Here's the drawing with two shaded views (mm, measured from the low corner). I have some questions. A direction names the side the tool comes from. Give positions to 0.01 mm unless a question says otherwise; leave off trailing zeros. Write each loop counter-clockwise with the first axis right and the second up, starting at its lowest first coordinate (ties: lowest second). Pieces come first, ordered by that corner, then holes. Notation, with made-up numbers: (1, -13.5) - (30, -13.5) arc R35 cw to (30, 22.5) - close; hole circle Ø10 at (0.5, 68). An arc over 180 degrees is marked (long way). Answer as a JSON object with one key per item and string values. Group by question number.
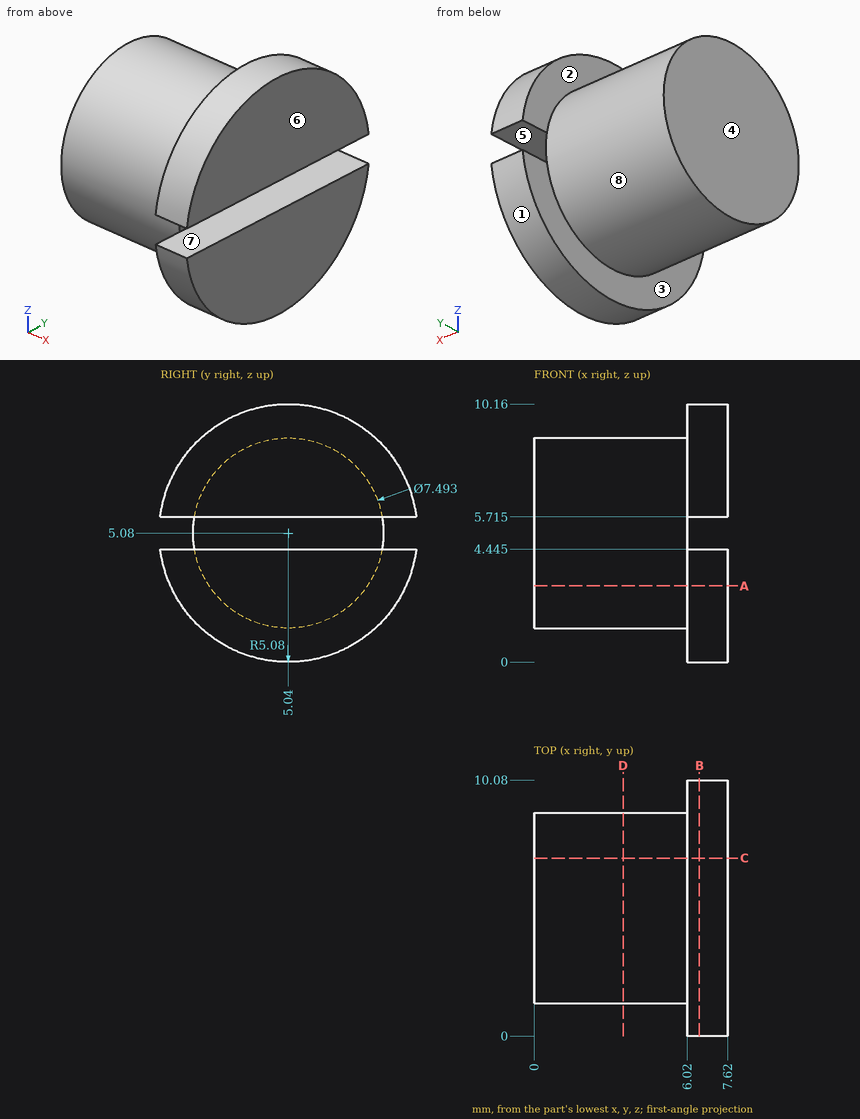
(1) I want a section at C-C, the plane y = 7. Please give me the cut outline in (x, z) (1 decimal), and give its area (3 significant figures).
(2) I want a section at D-D, the plane x = 3.5. Please give me the cut outline in (y, z), and give its area (3 significant figures).
(3) If we mould it in two halves opening along Z, with no side actions, what happens to the marked faces 6, 7 and 8? For each: +Z half, -Z half, draft (parallel to the pull), parting line (faces both ways), or undercut.
(4) Will these pins go through, and if not, where does the flat tip stop? P1, Ø3, axis at x = 6.5, y = 8, coming from the -Z side; P2, Ø3.5, axis at y = 7, z = 7.5, coming from the -X side; P3, Ø1.5, axis at x = 5, y = 4, coming from the -Z side (1 decimal); P4, Ø0.5, axis at x = 6.5, y = 6, coming from the -Z side.
(5) For the marked faces 1, 2, 3, 4 and 5, which set-ups out of +Z, -Z, +X, -X, +Y, -Y let a thin tool reach every point of the face, with its end or its side?
(6) I need wall thicknesses on L1, parallel to X at y = 2, z = 8.5; L2, parallel to Y at x = 5.75, z = 5 (1 decimal); L3, parallel to Z at x = 7, y = 7.5 (1 decimal). Which ranges of each line are inside material? Lowest first, please.
(7) I want a section at A-A, the plane z = 3. Please give me the cut outline in (x, y) (1 decimal).
(8) I want a section at B-B, the plane x = 6.5. Please give me the cut outline in (y, z) (1 decimal).
Entries:
{
 "1": {"outline": "(0, 1.9) - (6, 1.9) - (6, 0.4) - (7.6, 0.4) - (7.6, 4.4) - (6, 4.4) - (6, 5.7) - (7.6, 5.7) - (7.6, 9.8) - (6, 9.8) - (6, 8.3) - (0, 8.3) - close", "area": "51.4 mm^2"},
 "2": {"outline": "circle Ø7.49 at (5.04, 5.08)", "area": "44.1 mm^2"},
 "3": {"face 6": "draft", "face 7": "undercut", "face 8": "parting line"},
 "4": {"P1": "z = 0.21", "P2": "x = 0", "P3": "z = 1.3", "P4": "z = 0.05"},
 "5": {"face 1": "-Z, +X, -X", "face 2": "+Z, -X", "face 3": "-Z, -X", "face 4": "+Z, -Z, -X, +Y, -Y", "face 5": "+X, +Y, -Y"},
 "6": {"L1": "6.02 to 7.62", "L2": "1.3 to 8.8", "L3": "0.6 to 4.4, 5.7 to 9.5"},
 "7": {"outline": "(0, 1.9) - (6, 1.9) - (6, 0.4) - (7.6, 0.4) - (7.6, 9.7) - (6, 9.7) - (6, 8.2) - (0, 8.2) - close"},
 "8": {"outline": "(0, 4.4) arc R5.1 ccw to (10.1, 4.4) - close; (0, 5.7) - (10.1, 5.7) arc R5.1 ccw to start"}
}
